Here's how the part is built. I have some questions about the finished solid (model axes, mm). A direction names the side the tool comes from. Round coordinates to 2 decimals unless told otherwise and drop trailing zeros. Loops run counter-clockwise (first coordinate to the right, second up) from the corner with the lowest first, then second, coordinate; pieces in that order, holes last. Notation, with made-up numbers: M -25,77 L 22,77 A34 cw 22,108 Z; hole C 28,-17.5 d9. An arc over 180 degrees is marked long. Use a Markdown table: item, result.
from build123d import *

# Parameters (mm, degrees)
SKETCH_1_R              = 25
EXTRUDE_1_DEPTH         = 10
HOLE_WIZARD_M18_1_D     = 15.5
HOLE_WIZARD_M18_1_DEPTH = 43.5
HOLE_WIZARD_M18_1_TIP   = 4.656669797
HOLE_WIZARD_M6_1_D      = 5
HOLE_WIZARD_M6_1_DEPTH  = 5
HOLE_WIZARD_M6_1_TIP    = 1.502151548


with BuildPart() as part:
    # 草图1 → 凸台-拉伸1 (new body)
    with BuildSketch(Plane.XY):
        Circle(SKETCH_1_R)
    extrude(amount=EXTRUDE_1_DEPTH)

    # M18 螺纹孔1
    with Locations(Plane(origin=(0, 0, 0), x_dir=(-1, 0, 0), z_dir=(0, 0, -1))):
        with Locations((0, 0)):
            Hole(HOLE_WIZARD_M18_1_D / 2, depth=HOLE_WIZARD_M18_1_DEPTH)
            with Locations((0, 0, -(HOLE_WIZARD_M18_1_DEPTH + HOLE_WIZARD_M18_1_TIP / 2))):  # 118° drill point
                Cone(0, HOLE_WIZARD_M18_1_D / 2, HOLE_WIZARD_M18_1_TIP, mode=Mode.SUBTRACT)

    # M6 螺纹孔1
    with Locations(Plane(origin=(0, 0, 0), x_dir=(-1, 0, 0), z_dir=(0, 0, -1))):
        with Locations((0, 18), (-18, 0), (18, 0), (0, -18)):
            Hole(HOLE_WIZARD_M6_1_D / 2, depth=HOLE_WIZARD_M6_1_DEPTH)
            with Locations((0, 0, -(HOLE_WIZARD_M6_1_DEPTH + HOLE_WIZARD_M6_1_TIP / 2))):  # 118° drill point
                Cone(0, HOLE_WIZARD_M6_1_D / 2, HOLE_WIZARD_M6_1_TIP, mode=Mode.SUBTRACT)


solid = part.part
1. Imagine slicing it at D-D, the plane y = -4. Write out the boundary of the cut face in (x, z).
Answer sheet:
| item | result |
|---|---|
| outline | M -24.68,0 L -6.64,0 L -6.64,10 L -24.68,10 Z; M 6.64,0 L 24.68,0 L 24.68,10 L 6.64,10 Z |
2. Imagine slicing it at A-A, the plane z = 1.25. Write out the boundary of the cut face in (x, y).
Answer sheet:
| item | result |
|---|---|
| outline | C 0,0 d50; hole C -18,0 d5; hole C 0,0 d15.5; hole C 0,-18 d5; hole C 0,18 d5; hole C 18,0 d5 |
3. For pin 1 Ø3 at (x, y) = (0, -18) entering from -Z; pin 2 Ø4.5 at (x, y) = (18, 0) entering from -Z; pin 3 Ø6 at (y, z) = (-19, 6.5) entering from +X; pin 4 Ø14 at (x, y) = (0, 0) entering from +Z, each with a flat end and sliding along its axis, tell me the tip position at first contact or that it passes through.
Answer sheet:
| item | result |
|---|---|
| pin 1 | z = 5.6 |
| pin 2 | z = 5.15 |
| pin 3 | x = 19.21 |
| pin 4 | through |
4. We'd pull the mould along Y, two halves only. Please class faces 1 (the face through (-6, 6, 10)), 2 (the face through (-0.4, -18.17, 6.24)), 3 (the face through (23.846, 7.509, 4.93)), 4 (the face through (-18.4, -0.17, 6.24)): +Y half, -Y half, draft (parallel to the pull), parting line (faces both ways), or undercut.
Answer sheet:
| item | result |
|---|---|
| face 1 | draft |
| face 2 | undercut |
| face 3 | parting line |
| face 4 | undercut |
5. Which directions (+Z, -Z, +X, -X, +Y, -Y) give clear straight access to the entire face, cutting with the end or side of a thin tool? Please do faces 5 (the face through (-1.009, 7.684, 5.07)), 6 (the face through (15.5, 0.1, 2.5)).
Answer sheet:
| item | result |
|---|---|
| face 5 | +Z, -Z |
| face 6 | -Z |
6. Imagine slicing it at C-C, the plane z = 9. Write out the boundary of the cut face in (x, y), then the cut area to 3 significant figures.
Answer sheet:
| item | result |
|---|---|
| outline | C 0,0 d50; hole C 0,0 d15.5 |
| area | 1,770 mm2 |
7. I need wall thicknesses on probe 1 along Y at (x, z) = (0, 2.5); probe 2 along X at (y, z) = (-7, 8.5); probe 3 along X at (y, z) = (20, 2.5). Which ranges of each line are inside material? Lowest first, please. Write a range as from..to.
Answer sheet:
| item | result |
|---|---|
| probe 1 | -25..-20.5, -15.5..-7.75, 7.75..15.5, 20.5..25 |
| probe 2 | -24..-3.33, 3.33..24 |
| probe 3 | -15..-1.5, 1.5..15 |
8. Imagine slicing it at B-B, the plane y = 6. Write out the boundary of the cut face in (x, z), then the cut area to 3 significant figures.
Answer sheet:
| item | result |
|---|---|
| outline | M -24.27,0 L -4.91,0 L -4.91,10 L -24.27,10 Z; M 4.91,0 L 24.27,0 L 24.27,10 L 4.91,10 Z |
| area | 387 mm2 |
